```python
from build123d import *

# Parameters (mm, degrees)
F0_W      = 80
F0_H      = 600
F1_DEPTH  = 42
F2_W      = 80
F2_H      = 80
F3_DEPTH  = 14.5
F4_W      = 80
F4_H      = 80
F5_DEPTH  = 14.5
F7_DEPTH  = 14.5
F9_DEPTH  = 14.5
F11_DEPTH = 27.501
F13_DEPTH = 42.001
F15_DEPTH = 14.5
F17_DEPTH = 14.5


with BuildPart() as f1:
    # F0 (on Front) → F1 (new body)
    with BuildSketch(Plane.XZ):
        Rectangle(F0_W, F0_H)
    extrude(amount=F1_DEPTH)

    # F2 (on face) → F3 (cut)
    with BuildSketch(Plane.XZ.offset(42)):
        with Locations((0, 260)):
            Rectangle(F2_W, F2_H)
    extrude(amount=-F3_DEPTH, mode=Mode.SUBTRACT)

    # F4 (on face) → F5 (cut)
    with BuildSketch(Plane(origin=(0, 0, 0), x_dir=(-1, 0, 0), z_dir=(0, 1, 0))):
        with Locations((0, 260)):
            Rectangle(F4_W, F4_H)
    extrude(amount=-F5_DEPTH, mode=Mode.SUBTRACT)

    # F6 (on face) → F7 (cut, through all)
    with BuildSketch(Plane.XZ.offset(42)):
        Polygon((40, 220), (-40, 220), (40, 205.8938415433), align=None)
    extrude(amount=-F7_DEPTH, mode=Mode.SUBTRACT)

    # F8 (on face) → F9 (cut, through all)
    with BuildSketch(Plane(origin=(0, 0, 0), x_dir=(-1, 0, 0), z_dir=(0, 1, 0))):
        Polygon((-40, 205.8938415433), (40, 220), (-40, 220), align=None)
    extrude(amount=-F9_DEPTH, mode=Mode.SUBTRACT)

    # F10 (on face) → F11 (cut, through all)
    with BuildSketch(Plane.XZ.offset(27.5)):
        Polygon((-40, 300), (-40, 220), (-25.8938415433, 300), align=None)
        Polygon((40, 300), (-25.8938415433, 300), (40, 288.3811378734), align=None)
        Polygon((40, 288.3811378734), (25.8938415433, 208.3811378734), (40, 205.8938415433), align=None)
    extrude(amount=-F11_DEPTH, mode=Mode.SUBTRACT)

    # F12 (on face) → F13 (cut, through all)
    with BuildSketch(Plane.XZ.offset(42)):
        Polygon((-40, -300), (40, -300), (-40, -285.8938415433), align=None)
    extrude(amount=-F13_DEPTH, mode=Mode.SUBTRACT)

    # F14 (on face) → F15 (cut)
    with BuildSketch(Plane.XZ.offset(42)):
        Polygon((-40, -285.8938415433), (40, -300), (40, -218.7658710491), align=None)
    extrude(amount=-F15_DEPTH, mode=Mode.SUBTRACT)

    # F16 (on face) → F17 (cut)
    with BuildSketch(Plane(origin=(0, 0, 0), x_dir=(-1, 0, 0), z_dir=(0, 1, 0))):
        Polygon((-40, -218.7658710491), (-40, -300), (40, -285.8938415433), align=None)
    extrude(amount=-F17_DEPTH, mode=Mode.SUBTRACT)


solid = f1.part
```
Check sheet for the modelled part. Datum: model origin and axes. Units: mm. A direction names the side the tool comes from. Give positions to 0.01 mm unless a question says otherwise; leave off trailing zeros. Write each loop counter-clockwise with the first axis right and the second up, starting at its lowest first coordinate (ties: lowest second). Pieces come first, ordered by that corner, then holes.
Item 1: Gauge pin test, flat ends, axial feed: pin 1 (6 mm diameter, centred on x = 9, y = -26.5, fed in from +Z); pin 2 (24 mm diameter, centred on x = 4.5, z = -266, fed in from +Y); pin 3 (6 mm diameter, centred on x = 30, y = -32, fed in from -Z). Record the tip position at first contact, or that the pin passes through.
Item 2: Cross-section at B-B (x = -10.5). Enter the section's corners in (y, z), and give its area (3 significant figures).
Item 3: Access from +Z, -Z, +X, -X, +Y, -Y to the whole of each face (thin tool, end or side, straight path). Record for faces 1 (the face through (8, -27.5, -268)), 2 (the face through (-0.56, -7.15, -252.8)), 3 (the face through (6.592, -21.091, 294.272)), 4 (the face through (33.046, -21.091, 248.941)), 5 (the face through (40, -21, 6)).
Item 4: Cross-section at C-C (x = 15). Enter the section's corners in (y, z).
Item 5: Cross-section at A-A (y = -22). Enter the section's corners in (x, z).
Item 6: Scan lines: L1, parallel to Y at x = 10.5, z = -266.5; L2, parallel to Z at x = 29, y = -2; L3, parallel to Z at x = -15.5, y = -29. Record each from-to range of solid material in increasing order.
Report:
1. pin 1: stops at z = 294.38
1. pin 2: stops at y = -14.5
1. pin 3: stops at z = -229.67
2. outline: (-42, -261.14) - (-27.5, -261.14) - (-27.5, -291.1) - (-14.5, -291.1) - (-14.5, -261.14) - (0, -261.14) - (0, 214.8) - (-14.5, 214.8) - (-14.5, 297.29) - (-27.5, 297.29) - (-27.5, 214.8) - (-42, 214.8) - close
2. area: 21,500 mm2
3. face 1: -Z, +X, -Y
3. face 2: -Z, +X, +Y
3. face 3: +Z, +X, +Y, -Y
3. face 4: +X, +Y, -Y
3. face 5: +Z, -Z, +X, +Y, -Y
4. outline: (-42, -239.74) - (-27.5, -239.74) - (-27.5, -295.59) - (-14.5, -295.59) - (-14.5, -239.74) - (0, -239.74) - (0, 210.3) - (-14.5, 210.3) - (-14.5, 292.79) - (-27.5, 292.79) - (-27.5, 210.3) - (-42, 210.3) - close
5. outline: (-40, -285.89) - (40, -300) - (40, 205.89) - (25.89, 208.38) - (40, 288.38) - (-25.89, 300) - (-40, 220) - close
6. L1: y = -27.5 to -14.5
6. L2: z = -228 to 207.83
6. L3: z = -265.34 to 215.68
